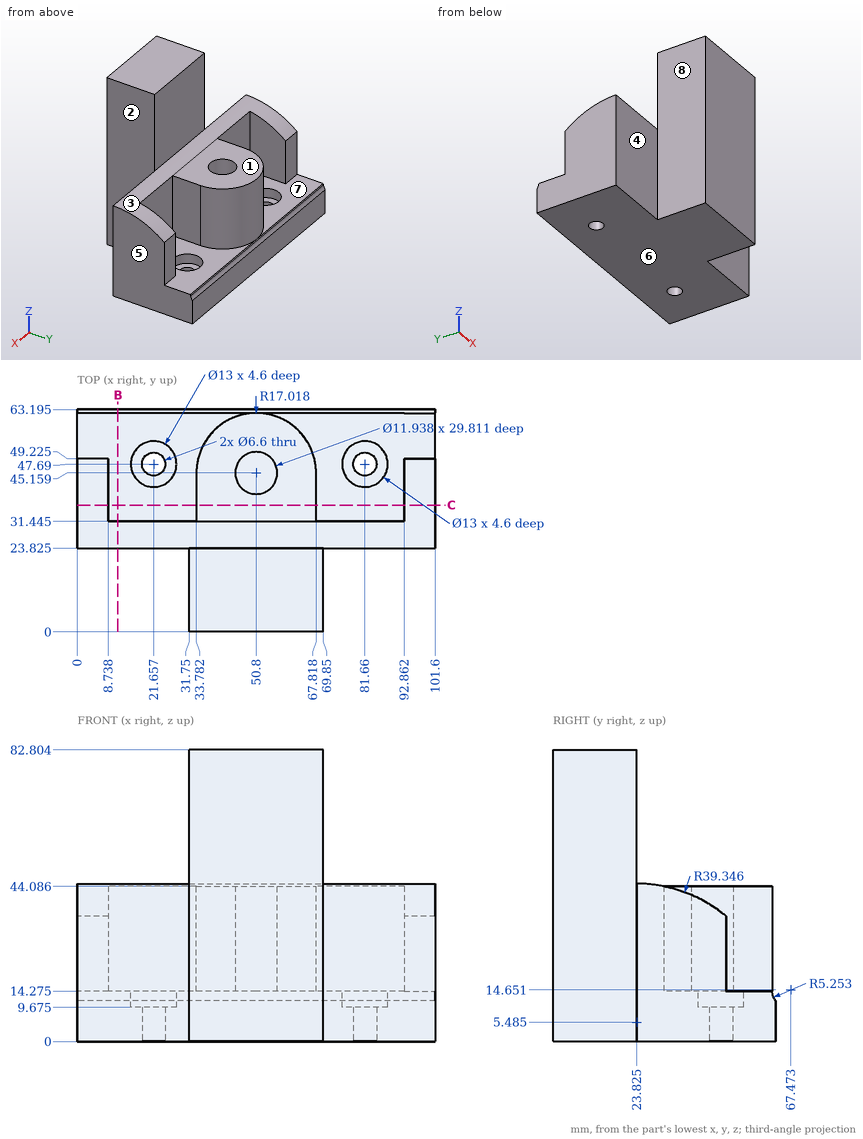
Can you work these out from the drawing? Everything is in mm from the part's minimum corner. A direction names the side the tool comes from. Round coordinates to 2 decimals unless told otherwise and drop trailing zeros. Order: outer loops, then holes, each group sorted by start corner. A loop starts at its lowest first (then second) coordinate and runs counter-clockwise, first axis right, second up. Notation, with made-up numbers: M 11.5,41.25 L 24.5,41.25 A29 cw 24.5,75.25 Z; hole C 47.5,37.5 d5. An arc over 180 degrees is marked long. Answer as CSV lines item,"result".
Item 1: For pin 1 (4 mm diameter, centred on x = 18.5, y = 50, fed in from +Z) (1 decimal); pin 2 (4.5 mm diameter, centred on x = 5.5, z = 23.5, fed in from +Y) (1 decimal); pin 3 (16 mm diameter, centred on x = 89, z = 20.5, fed in from -Y) (1 decimal), each with a flat end and sliding along its axis, tell me the tip position at first contact or that it passes through.
From the geometry:
pin 1,"z = 9.7"
pin 2,"y = 49.2"
pin 3,"y = 23.8"
Item 2: Which directions (+Z, -Z, +X, -X, +Y, -Y) give clear straight access to the entire face, cutting with the end or side of a thin tool? Please do the marked faces 1, 2, 3 and 4.
From the geometry:
face 1,"+Z, +X, -X, +Y"
face 2,"+Z, -Z, +X, -Y"
face 3,"+Z, +Y"
face 4,"+Z, -Z, -X, -Y"
Item 3: Imagine slicing it at C-C on y = 36. List the corners of the cut face in (x, z) for me (1 decimal).
From the geometry:
outline,"M 0,0 L 101.6,0 L 101.6,42.9 L 92.9,42.9 L 92.9,14.3 L 67.8,14.3 L 67.8,44.1 L 33.8,44.1 L 33.8,14.3 L 8.7,14.3 L 8.7,42.9 L 0,42.9 Z"
Item 4: Please list where these lines run through material, in increasing order: L1, parallel to X at y = 38, z = 34.5; L2, parallel to X at y = 43.5, z = 34 (1 decimal); L3, parallel to Y at x = 50.8, z = 37.25. Write a range as [from, to].
From the geometry:
L1,"[0, 8.74], [33.78, 67.82], [92.86, 101.6]"
L2,"[0, 8.7], [33.8, 45.1], [56.5, 67.8], [92.9, 101.6]"
L3,"[0, 39.19], [51.13, 62.18]"
Item 5: We'd pull the mould along X, two halves only. Please class the marked faces 5, 6, 7 and 8: +X half, -X half, draft (parallel to the pull), parting line (faces both ways), or undercut.
From the geometry:
face 5,"+X half"
face 6,"draft"
face 7,"undercut"
face 8,"-X half"
Item 6: Imagine slicing it at B-B on x = 11.5. List the corners of the cut face in (y, z) for me (1 decimal), and give its area (3 significant figures).
From the geometry:
outline,"M 23.8,0 L 63.2,0 L 63.2,11.6 A5.3 cw 62.3,13.6 A39.3 ccw 62.2,14.3 L 31.4,14.3 L 31.4,44.1 A39.3 ccw 23.8,44.8 Z"
area,"791 mm2"
